from build123d import *

# Parameters (mm, degrees)
F0_R     = 35
F1_DEPTH = 15
F2_W     = 35
F2_H     = 35
F3_DEPTH = 20
F4_W     = 18.214288
F4_H     = 20
F5_DEPTH = 30


with BuildPart() as f1:
    # F0 (on Top) → F1 (new body)
    with BuildSketch(Plane.XY):
        Circle(F0_R)
    extrude(amount=F1_DEPTH)

    # F2 (on face) → F3 (join)
    with BuildSketch(Plane.XY.offset(15)):
        Rectangle(F2_W, F2_H)
    extrude(amount=F3_DEPTH)

    # F4 (on face) → F5 (join)
    with BuildSketch(Plane.XY.offset(35)):
        Rectangle(F4_W, F4_H)
    extrude(amount=F5_DEPTH)


solid = f1.part
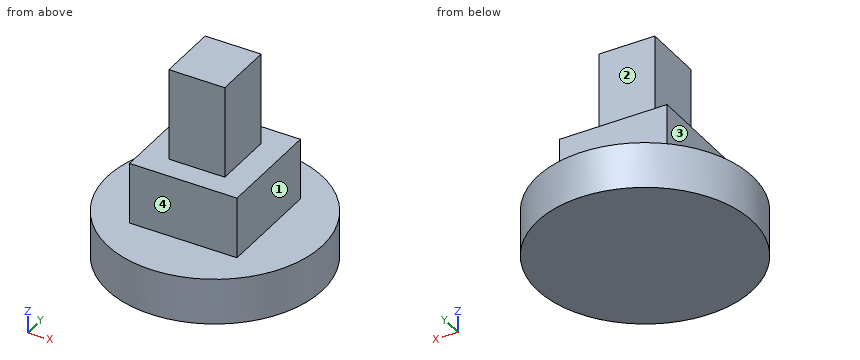
Can you work these out from the model? Positions are in its coordinate system, mm. Face numbers are marked on the shaded views. A direction names the side the tool comes from. Give positions to 0.01 mm unless a question says otherwise; leave off trailing zeros. Write each loop counter-clockwise with the first axis right and the second up, starting at its lowest first coordinate (ties: lowest second). Pieces come first, ordered by that corner, then holes. Notation, with made-up numbers: M 15,88 L 36,88 A19 ccw 36,95 Z; hole C 29,76.5 d2. An arc over 180 degrees is marked long. Answer in a Markdown table with one row per item. Add a question column.
Item 1: Imagine slicing it at A-A, the plane x = 0. Write out the boundary of the cut face in (y, z), plus the area to 3 significant figures.
Item 2: On a 3-axis mill with a long thin cutter (end or side, diameter ignored), from which of +Z, -Z, +X, -X, +Y, -Y can I reach the whole of each face in a straight line? I mean the marked faces 1, 2, 3 and 4. Say none if no direction works.
Item 3: Imagine slicing it at B-B, the plane y = 0. Write out the boundary of the cut face in (x, z).
Item 4: Please list where these lines run through material, in increasing order: L1, parallel to X at y = -6, z = 19; L2, parallel to Z at x = -7, y = 10.5; L3, parallel to Z at x = 15, y = 27.
Item 5: For pin 1 Ø4 at (x, y) = (25.5, 5) entering from +Z; pin 2 Ø8 at (y, z) = (6.5, 58) entering from +X; pin 3 Ø6 at (y, z) = (-0.5, 55) entering from -X; pin 4 Ø1 at (x, y) = (15.5, 8) entering from -Z, each with a flat end and sliding along its axis, tell me the tip position at first contact or that it passes through.
Item 6: Imagine slicing it at D-D, the plane x = -11.5. Write out the boundary of the cut face in (y, z), plus the area to 3 significant figures.
Item 7: Imagine slicing it at C-C, the plane z = 52.5. Write out the boundary of the cut face in (x, y).
Evaluation:
| question | item | result |
|---|---|---|
| 1 | outline | M -35,0 L 35,0 L 35,15 L 17.5,15 L 17.5,35 L 10,35 L 10,65 L -10,65 L -10,35 L -17.5,35 L -17.5,15 L -35,15 Z |
| 1 | area | 2,350 mm² |
| 2 | face 1 | +Z, +X, +Y, -Y |
| 2 | face 2 | +Z, +X, -X, +Y |
| 2 | face 3 | +Z, -X, +Y, -Y |
| 2 | face 4 | +Z, +X, -X, -Y |
| 3 | outline | M -35,0 L 35,0 L 35,15 L 17.5,15 L 17.5,35 L 9.11,35 L 9.11,65 L -9.11,65 L -9.11,35 L -17.5,35 L -17.5,15 L -35,15 Z |
| 4 | L1 | x = -17.5 to 17.5 |
| 4 | L2 | z = 0 to 35 |
| 4 | L3 | z = 0 to 15 |
| 5 | pin 1 | stops at z = 15 |
| 5 | pin 2 | stops at x = 9.11 |
| 5 | pin 3 | stops at x = -9.11 |
| 5 | pin 4 | stops at z = 0 |
| 6 | outline | M -33.06,0 L 33.06,0 L 33.06,15 L 17.5,15 L 17.5,35 L -17.5,35 L -17.5,15 L -33.06,15 Z |
| 6 | area | 1,690 mm² |
| 7 | outline | M -9.11,-10 L 9.11,-10 L 9.11,10 L -9.11,10 Z |
